```python
from build123d import *

# Parameters (mm, degrees)
BOSS_EXTRUDE1_DEPTH = 25
CUT_EXTRUDE1_DEPTH  = 9
FILLET1_R           = 7
SKETCH4_R           = 4
CUT_EXTRUDE2_DEPTH  = 9


with BuildPart() as part:
    # Sketch2 → Boss-Extrude1 (new, symmetric)
    with BuildSketch(Plane.XY):
        with BuildLine():
            Line((23, 0), (57, 0))
            Line((57, 0), (57, 42))
            Line((57, 42), (48, 42))
            Line((48, 42), (48, 11))
            ThreePointArc((48, 11), (47.414213562, 9.585786438), (46, 9))
            Line((46, 9), (32.171415884, 9))
            ThreePointArc((32.171415884, 9), (31.008255888, 9.373021566), (30.278979656, 10.352941176))
            ThreePointArc((30.278979656, 10.352941176), (0, 32), (-30.278979656, 10.352941176))
            ThreePointArc((-30.278979656, 10.352941176), (-31.008255888, 9.373021566), (-32.171415884, 9))
            Line((-32.171415884, 9), (-58, 9))
            Line((-58, 9), (-58, 0))
            Line((-58, 0), (-23, 0))
            ThreePointArc((-23, 0), (0, 23), (23, 0))
        make_face()
    extrude(amount=BOSS_EXTRUDE1_DEPTH, both=True)

    # Sketch3 → Cut-Extrude1 (cut)
    with BuildSketch(Plane(origin=(57, 0, 0), x_dir=(0, 0, -1), z_dir=(1, 0, 0))):
        with BuildLine():
            Line((-6, 24), (-6, 42))
            Line((-6, 42), (6, 42))
            Line((6, 42), (6, 24))
            ThreePointArc((6, 24), (0, 18), (-6, 24))
        make_face()
    extrude(amount=-CUT_EXTRUDE1_DEPTH, mode=Mode.SUBTRACT)

    # Fillet1
    fillet1_edges = [part.edges().sort_by_distance(p)[0] for p in [
        (-58, 4.5, -25),
        (52.5, 42, -25),
        (52.5, 42, 25),
        (-58, 4.5, 25),
    ]]
    fillet(fillet1_edges, radius=FILLET1_R)

    # Sketch4 → Cut-Extrude2 (cut)
    with BuildSketch(Plane(origin=(0, 9, 0), x_dir=(1, 0, 0), z_dir=(0, 1, 0))):
        with Locations(Location((-51, 18, 0), (0, 0, 270))):
            Circle(SKETCH4_R)
        with Locations(Location((-51, -18, 0), (0, 0, 270))):
            Circle(SKETCH4_R)
    extrude(amount=-CUT_EXTRUDE2_DEPTH, mode=Mode.SUBTRACT)


solid = part.part
```
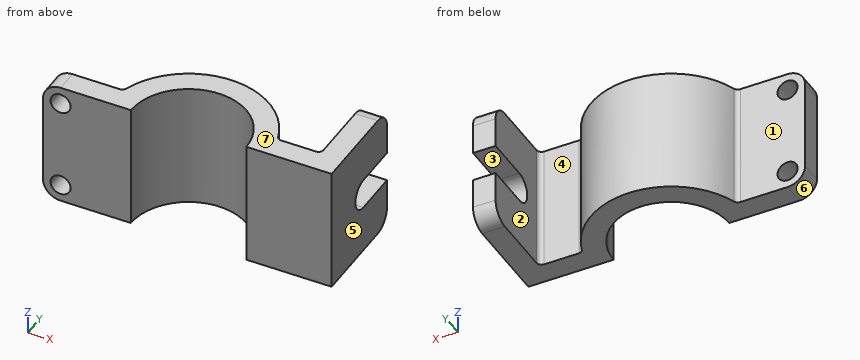
Source: CAD feature listing. Evaluate the final solid. Frame: model axes, mm. Face numbers are marked on the shaded views. A direction names the side the tool comes from. Round coordinates to 2 decimals unless told otherwise and drop trailing zeros. Loops run counter-clockwise (first coordinate to the right, second up) from the corner with the lowest first, then second, coordinate; pieces in that order, holes last. Notation, with made-up numbers: M -0.75,-31.5 L 20.25,-31.5 A28 cw 20.25,3.5 Z; hole C 88,3.25 d1. An arc over 180 degrees is marked long. Use a Markdown table: item, result. Add a question column.
1. Reachability of the marked faces 1, 2 and 3 from +Z, -Z, +X, -X, +Y, -Y: full face, straight path, thin tool, end or side. Return the list, or none.
2. Line query: line 1 (X direction, y = 3, z = -18); line 2 (X direction, y = 17.5, z = -3.5); line 3 (X direction, y = 34, z = -11). Output: solid intervals per line, ascending.
3. Section query B-B on z = -8. Return the cut outline in (x, y), then the cut area to 3 significant figures.
4. Section query C-C on y = 38. Return the cut outline in (x, z).
5. Section query D-D on z = 0. Return the cut outline in (x, y).
6. Section query A-A on y = 3.5. Return the cut outline in (x, z).
7. Mould query, pull axis X, two halves, no side actions, for the marked faces 4, 5, 6 and 7. Classes: pulls with the +X half, pulls with the -X half, needs draft (parallel to the pull), parting line crosses it, or undercut.
8. Contact query for flat-ended pins moving along their axis: P1, Ø12, axis at x = -13, z = 2, coming from the +Y side (3 decimals); P2, Ø7, axis at x = 40.5, z = 8.5, coming from the +Y side; P3, Ø2, axis at x = -14.5, z = -16, coming from the -Y side; P4, Ø10, axis at x = 52.5, y = 37.5, coming from the -Z side. Output: stop coordinate, or through.
Reported:
| question | item | result |
|---|---|---|
| 1 | face 1 | +Z, -Z, -X, +Y |
| 1 | face 2 | +Z, -Z, +Y |
| 1 | face 3 | +X, +Y |
| 2 | line 1 | x = -58 to -55, -47 to -22.8, 22.8 to 57 |
| 2 | line 2 | x = -26.79 to -14.92, 14.92 to 26.79, 48 to 57 |
| 2 | line 3 | x = 48 to 57 |
| 3 | outline | M -58,0 L -23,0 A23 cw 23,0 L 57,0 L 57,42 L 48,42 L 48,11 A2 cw 46,9 L 32.17,9 A2 cw 30.28,10.35 A32 ccw -30.28,10.35 A2 cw -32.17,9 L -58,9 Z |
| 3 | area | 1,540 mm² |
| 4 | outline | M 48,-24.32 L 57,-24.32 L 57,-6 L 48,-6 Z; M 48,6 L 57,6 L 57,24.32 L 48,24.32 Z |
| 5 | outline | M -58,0 L -23,0 A23 cw 23,0 L 57,0 L 57,18 L 48,18 L 48,11 A2 cw 46,9 L 32.17,9 A2 cw 30.28,10.35 A32 ccw -30.28,10.35 A2 cw -32.17,9 L -58,9 Z |
| 6 | outline | M -58,-18 A7 ccw -51,-25 L -22.73,-25 L -22.73,25 L -51,25 A7 ccw -58,18 Z; M 22.73,-25 L 57,-25 L 57,25 L 22.73,25 Z; hole C -51,-18 d8; hole C -51,18 d8 |
| 7 | face 4 | undercut |
| 7 | face 5 | pulls with the +X half |
| 7 | face 6 | pulls with the -X half |
| 7 | face 7 | needs draft |
| 8 | P1 | stops at y = 31.225 |
| 8 | P2 | stops at y = 9 |
| 8 | P3 | stops at y = 16.99 |
| 8 | P4 | stops at z = -25 |
